Here's how the part is built. I have some questions about the finished solid (model axes, mm). Round coordinates to 2 decimals unless told otherwise and drop trailing zeros. Loops run counter-clockwise (first coordinate to the right, second up) from the corner with the lowest first, then second, coordinate; pieces in that order, holes last. Notation, with made-up numbers: M 16.5,76 L 43.5,76 A15 cw 43.5,87 Z; hole C 67.25,-14 d10. An arc over 180 degrees is marked long. Answer as a JSON object with one key per item and string values.
from build123d import *

# Parameters (mm, degrees)
SKETCH_1_W      = 65
SKETCH_1_H      = 65
SKETCH_1_R      = 1.6
EXTRUDE_1_DEPTH = 1.5


with BuildPart() as part:
    # Эскиз1 → Бобышка-Вытянуть1 (new body)
    # profile 1 of 3: a face of its own
    with BuildSketch(Plane(origin=(0, 0, 0), x_dir=(1, 0, 0), z_dir=(0, 1, 0))):
        with BuildLine():
            Line((-32.5, -32.5), (32.5, -32.5))
            ThreePointArc((32.5, -32.5), (0, -46), (-32.5, -32.5))
        make_face()
    # profile 2 of 3: a face of its own
    with BuildSketch(Plane(origin=(0, 0, 0), x_dir=(1, 0, 0), z_dir=(0, 1, 0))):
        Rectangle(SKETCH_1_W, SKETCH_1_H)
        with Locations(Location((-28, -30, 0), (0, 0, 270))):
            Circle(SKETCH_1_R, mode=Mode.SUBTRACT)
        with Locations(Location((-28, 30, 0), (0, 0, 270))):
            Circle(SKETCH_1_R, mode=Mode.SUBTRACT)
        with Locations(Location((28, 30, 0), (0, 0, 270))):
            Circle(SKETCH_1_R, mode=Mode.SUBTRACT)
        with Locations(Location((28, -30, 0), (0, 0, 270))):
            Circle(SKETCH_1_R, mode=Mode.SUBTRACT)
    # profile 3 of 3: a face of its own
    with BuildSketch(Plane(origin=(0, 0, 0), x_dir=(1, 0, 0), z_dir=(0, 1, 0))):
        with BuildLine():
            ThreePointArc((-32.5, 32.5), (0, 46), (32.5, 32.5))
            Line((32.5, 32.5), (-32.5, 32.5))
        make_face()
    extrude(amount=EXTRUDE_1_DEPTH)


solid = part.part
Item 1: I want a section at A-A on z = -30. List the corners of the cut face in (x, y) for me, plus the area to 3 significant figures.
Solution:
{"outline": "M -32.5,0 L -29.6,0 L -29.6,1.5 L -32.5,1.5 Z; M -26.4,0 L 26.4,0 L 26.4,1.5 L -26.4,1.5 Z; M 29.6,0 L 32.5,0 L 32.5,1.5 L 29.6,1.5 Z", "area": "87.9 mm2"}
Item 2: If I drill on L1, parallel to X at y = 1, z = -30; L2, parallel to Z at x = 28.5, y = 0.1; L3, parallel to Z at x = 0.5, y = 0.65, over which ranges is the centre line in solid material (lowest first)? Write a range as from..to.
Solution:
{"L1": "x = -32.5..-29.6, -26.4..26.4, 29.6..32.5", "L2": "z = -36.07..-31.52, -28.48..28.48, 31.52..36.07", "L3": "z = -46..46"}
Item 3: I want a section at C-C on x = -28. List the corners of the cut face in (y, z) for me.
Solution:
{"outline": "M 0,-36.46 L 1.5,-36.46 L 1.5,-31.6 L 0,-31.6 Z; M 0,-28.4 L 1.5,-28.4 L 1.5,28.4 L 0,28.4 Z; M 0,31.6 L 1.5,31.6 L 1.5,36.46 L 0,36.46 Z"}
Item 4: We'd pull the mould along Z, two halves only. Please class faces 1 (the face through (0, 1.5, -1)), 2 (the face through (0.506, 0.74, 45.997)), 3 (the face through (-0.506, 0.74, -45.997)), 4 (the face through (-26.92, 0.74, -31.18)): +Z half, -Z half, draft (parallel to the pull), parting line (faces both ways), or undercut.
Solution:
{"face 1": "draft", "face 2": "+Z half", "face 3": "-Z half", "face 4": "undercut"}
Item 5: I want a section at B-B on y = 0.3. List the corners of the cut face in (x, z) for me.
Solution:
{"outline": "M -32.5,-32.5 A45.87 ccw 32.5,-32.5 L 32.5,32.5 A45.87 ccw -32.5,32.5 Z; hole C -28,-30 d3.2; hole C -28,30 d3.2; hole C 28,-30 d3.2; hole C 28,30 d3.2"}
Item 6: I want a section at D-D on x = -16.5. List the corners of the cut face in (y, z) for me.
Solution:
{"outline": "M 0,-42.93 L 1.5,-42.93 L 1.5,42.93 L 0,42.93 Z"}
